```python
from build123d import *

# Parameters (mm, degrees)
SCHIZZO2_W                   = 523
SCHIZZO2_H                   = 513
ESTRUSIONE_ESTRUSIONE2_DEPTH = 130
SVUOTA1_T                    = -5
TAGLIO_ESTRUSIONE2_REACH     = 610.702
ESTRUSIONE_ESTRUSIONE3_DEPTH = 523
TAGLIO_ESTRUSIONE3_DEPTH     = 10
SCHIZZO5_W                   = 5
SCHIZZO5_H                   = 513
ESTRUSIONE_ESTRUSIONE5_DEPTH = 30
TAGLIO_ESTRUSIONE4_REACH     = 610.702


with BuildPart() as part:
    # Schizzo2 → Estrusione-Estrusione2 (new body)
    with BuildSketch(Plane.XY):
        with Locations((26.5, 26.5)):
            Rectangle(SCHIZZO2_W, SCHIZZO2_H)
    extrude(amount=ESTRUSIONE_ESTRUSIONE2_DEPTH)

    # Svuota1
    svuota1_openings = [part.faces().sort_by_distance(p)[0] for p in [
        (26.5, 26.5, 0),
    ]]
    offset(amount=SVUOTA1_T, openings=svuota1_openings, kind=Kind.INTERSECTION)

    # Taglio-Estrusione2: up to this face of the body (flat: up to its plane)
    taglio_estrusione2_end = Plane(part.part.faces().sort_by_distance((-235, 26.5, 65))[0])
    # Schizzo3 → Taglio-Estrusione2 (cut, up to the picked face)
    with BuildSketch(Plane(origin=(288, 0, 0), x_dir=(0, 0, -1), z_dir=(1, 0, 0)), mode=Mode.PRIVATE) as taglio_estrusione2_sk1:
        Polygon((-30, -230), (-130, -130), (-130, -230), align=None)
    taglio_estrusione2_tool1 = split(extrude(taglio_estrusione2_sk1.sketch, amount=-TAGLIO_ESTRUSIONE2_REACH, mode=Mode.PRIVATE), bisect_by=taglio_estrusione2_end, keep=Keep.BOTH, mode=Mode.PRIVATE)
    add(taglio_estrusione2_tool1.solids().sort_by(Axis((288, -196.666667, 96.666667), (-1, 0, 0)))[0], mode=Mode.SUBTRACT)

    # Schizzo3<4> → Estrusione-Estrusione3 (add)
    with BuildSketch(Plane(origin=(288, 0, 0), x_dir=(0, 0, -1), z_dir=(1, 0, 0))):
        Polygon((-130, -122.928932188), (-130, -130), (-30, -230), (-22.928932188, -230), align=None)
    extrude(amount=-ESTRUSIONE_ESTRUSIONE3_DEPTH)

    # Schizzo4 → Taglio-Estrusione3 (cut)
    with BuildSketch(Plane(origin=(0, 283, 0), x_dir=(1, 0, 0), z_dir=(0, 1, 0))):
        Polygon((-213.5, -65), (266.5, -65), (266.5, -45), (36.5, -45), (36.5, 0), (16.5, 0), (16.5, -45), (-213.5, -45), align=None)
    extrude(amount=-TAGLIO_ESTRUSIONE3_DEPTH, mode=Mode.SUBTRACT)

    # Schizzo5 → Estrusione-Estrusione5 (add)
    with BuildSketch(Plane.XY):
        with Locations((285.5, 26.5)):
            Rectangle(SCHIZZO5_W, SCHIZZO5_H)
        with Locations((-232.5, 26.5)):
            Rectangle(SCHIZZO5_W, SCHIZZO5_H)
    extrude(amount=-ESTRUSIONE_ESTRUSIONE5_DEPTH)

    # Taglio-Estrusione4: up to this face of the body (flat: up to its plane)
    taglio_estrusione4_end = Plane(part.part.faces().sort_by_distance((288, 40.976301678, 46.972842069))[0])
    # Schizzo6 → Taglio-Estrusione4 (cut, up to the picked face)
    with BuildSketch(Plane.ZY.offset(235), mode=Mode.PRIVATE) as taglio_estrusione4_sk1:
        with BuildLine():
            Line((-15, 133.05), (-30, 133.05))
            Line((-30, 133.05), (-30, 126.95))
            Line((-30, 126.95), (-15, 126.95))
            ThreePointArc((-15, 126.95), (-11.95, 130), (-15, 133.05))
        make_face()
    taglio_estrusione4_tool1 = split(extrude(taglio_estrusione4_sk1.sketch, amount=-TAGLIO_ESTRUSIONE4_REACH, mode=Mode.PRIVATE), bisect_by=taglio_estrusione4_end, keep=Keep.BOTH, mode=Mode.PRIVATE)
    # Schizzo6 → Taglio-Estrusione4 (cut, up to the picked face)
    with BuildSketch(Plane.ZY.offset(235), mode=Mode.PRIVATE) as taglio_estrusione4_sk2:
        with BuildLine():
            Line((-30, -133.05), (-30, -126.95))
            Line((-30, -126.95), (-15, -126.95))
            ThreePointArc((-15, -126.95), (-11.95, -130), (-15, -133.05))
            Line((-15, -133.05), (-30, -133.05))
        make_face()
    taglio_estrusione4_tool2 = split(extrude(taglio_estrusione4_sk2.sketch, amount=-TAGLIO_ESTRUSIONE4_REACH, mode=Mode.PRIVATE), bisect_by=taglio_estrusione4_end, keep=Keep.BOTH, mode=Mode.PRIVATE)
    add(taglio_estrusione4_tool1.solids().sort_by(Axis((-235, 130, -21.288948), (1, 0, 0)))[0], mode=Mode.SUBTRACT)
    add(taglio_estrusione4_tool2.solids().sort_by(Axis((-235, -130, -21.288948), (1, 0, 0)))[0], mode=Mode.SUBTRACT)


solid = part.part
```
Work out the finished part from the listing and answer in its coordinate system (mm). A direction names the side the tool comes from. Give positions to 0.01 mm unless a question says otherwise; leave off trailing zeros. Write each loop counter-clockwise with the first axis right and the second up, starting at its lowest first coordinate (ties: lowest second). Pieces come first, ordered by that corner, then holes.
(1) The part is cut by section B-B on y = 214. Write down the section's boundary in (x, z), plus the area to 4 significant figures.
Final values:
outline: (-235, -30) - (-230, -30) - (-230, 125) - (283, 125) - (283, -30) - (288, -30) - (288, 130) - (-235, 130) - close
area: 4,165 mm2
(2) The mould has two halves that part along X. Classify faces 1 (the flat face through (23, 79, 130)), 2 (the flat face through (288, 23, 51)), 3 (the flat face through (-235, 23, 49)), 4 (the flat face through (23, -225, 14)): pulls with the +X half, pulls with the -X half, needs draft (parallel to the pull), parting line crosses it, or undercut.
Final values:
face 1: needs draft
face 2: pulls with the +X half
face 3: pulls with the -X half
face 4: undercut
(3) The part is cut by section C-C on z = 12. Write down the section's boundary in (x, y), plus the area to 3 significant figures.
Final values:
outline: (-235, -230) - (288, -230) - (288, 283) - (36.5, 283) - (36.5, 278) - (283, 278) - (283, -225) - (-230, -225) - (-230, 278) - (16.5, 278) - (16.5, 283) - (-235, 283) - close
area: 10,200 mm2
(4) Straight lines are drawn through the part: line 1 (X direction, y = 113.5, z = 53.5); line 2 (Y direction, x = 208.5, z = 16.5); line 3 (Z direction, x = 198, y = 45). For each, find the intervals that lie inside material, in ascending order.
Final values:
line 1: x = -235 to -230, 283 to 288
line 2: y = -230 to -225, 278 to 283
line 3: z = 125 to 130
(5) The part is cut by section D-D on z = 71.5. Write down the section's boundary in (x, y).
Final values:
outline: (-235, -188.5) - (288, -188.5) - (288, 283) - (-235, 283) - close; hole (-230, -181.43) - (283, -181.43) - (283, 278) - (-230, 278) - close
(6) Which of the six approach directions +Z, -Z, +X, -X, +Y, -Y give full straight-line access (tool end or side, diameter ignored) to faces 5 (the flat face through (23, 283, 69)), 6 (the flat face through (23, 278, 76))?
Final values:
face 5: +Z, -Z, +X, -X, +Y
face 6: -Z
(7) Flat-ended cylindrical pins translate along their axes: pin 1 Ø4 at (x, z) = (73.5, 56) entering from +Y; pin 2 Ø5.5 at (x, y) = (128.5, 280) entering from -Z; pin 3 Ø6 at (x, y) = (-61.5, -137.5) entering from -Z. Find the tip coordinate at first contact, or state that the pin passes through.
Final values:
pin 1: stops at y = -194.93
pin 2: stops at z = 0
pin 3: stops at z = 112.43
(8) The part is cut by section A-A on x = -59. Write down the section's boundary in (y, z).
Final values:
outline: (-230, 0) - (-225, 0) - (-225, 27.93) - (-127.93, 125) - (278, 125) - (278, 65) - (283, 65) - (283, 130) - (-130, 130) - (-230, 30) - close; (278, 0) - (283, 0) - (283, 45) - (278, 45) - close
